The model under review builds one solid part; all positions refer to its coordinate system, in mm. Face numbers are marked on the shaded views. Round coordinates to 2 decimals unless told otherwise and drop trailing zeros. Write each loop counter-clockwise with the first axis right and the second up, starting at its lowest first coordinate (ties: lowest second). Pieces come first, ordered by that corner, then holes. Notation, with made-up numbers: (69.25, 74.5) -> (128.25, 74.5) arc R29 cw to (128.25, 101.5) -> close; hole circle Ø10 at (27, -10.5). An arc over 180 degrees is marked (long way). Use CSV: the item, a comma, the result in double quotes. Start each with the question number.
1) For pin 1 Ø12 at (y, z) = (88.5, 2) entering from -X; pin 2 Ø12 at (y, z) = (55.5, -14.5) entering from +X; pin 3 Ø10.5 at (x, z) = (40.05, -23.12) entering from -Y; pin 4 Ø12 at (y, z) = (107.5, -38.5) entering from -X, all flat-tipped, find the tip position at first contact; note any pin that passes through.
2) Take a section at C-C, the plane y = 70.5. Give the boundary of the cut face in (x, z), then the cut area to 3 significant figures.
3) Wall thickness on probe 1 along Y at (x, z) = (-24.5, -34); probe 2 along X at (y, z) = (87, 0); probe 3 along Z at (x, y) = (-36.5, 58): over which ranges is each line inside the solid? List them lowest first. Write a range as [from, to].
4) Mouldability with a two-part tool opening along Z and no side actions: class the marked faces 1, 2, 3 and 4 as released by +Z, released by -Z, zero draft, split by the parting line, or undercut.
from build123d import *

# Parameters (mm, degrees)
SKETCH1_R                       = 52.5
SKETCH1_R_2                     = 40
BOSS_EXTRUDE1_DEPTH             = 150
SKETCH7_R                       = 42.5
YLIN_URA_DEPTH                  = 3.6
SKETCH8_R                       = 42.5
TOKA_YLIN_URA_DEPTH             = 3.6
CUT_EXTRUDE5_START              = -3.6
SKETCH10_R                      = 42.5
CUT_EXTRUDE5_DEPTH              = 3.6
F_8_0MM_DOWEL_HOLE1_D           = 8
F_8_0MM_DOWEL_HOLE1_DEPTH       = 22.596557524
F_8_0MM_DOWEL_HOLE1_CSINK_D     = 8.05
F_8_0MM_DOWEL_HOLE1_CSINK_ANGLE = 90
F_8_0MM_DOWEL_HOLE1_TIP         = 2.403442476


with BuildPart() as part:
    # Sketch1 → Boss-Extrude1 (new body)
    with BuildSketch(Plane(origin=(0, 0, 0), x_dir=(1, 0, 0), z_dir=(0, 1, 0))):
        with Locations(Location((0, 0, 0), (0, 0, 270))):
            Circle(SKETCH1_R)
        with Locations(Location((0, 0, 0), (0, 0, 270))):
            Circle(SKETCH1_R_2, mode=Mode.SUBTRACT)
    extrude(amount=BOSS_EXTRUDE1_DEPTH)

    # Sketch7 → Ylin ura (cut)
    with BuildSketch(Plane(origin=(0, 135, 0), x_dir=(1, 0, 0), z_dir=(0, 1, 0))):
        with Locations(Location((0, 0, 0), (0, 0, 270))):
            Circle(SKETCH7_R)
    extrude(amount=-YLIN_URA_DEPTH, mode=Mode.SUBTRACT)

    # Sketch8 → Toka ylin ura (cut)
    with BuildSketch(Plane(origin=(0, 109.9, 0), x_dir=(1, 0, 0), z_dir=(0, 1, 0))):
        with Locations(Location((0, 0, 0), (0, 0, 270))):
            Circle(SKETCH8_R)
    extrude(amount=-TOKA_YLIN_URA_DEPTH, mode=Mode.SUBTRACT)

    # Sketch10 → Cut-Extrude5 (cut)
    with BuildSketch(Plane(origin=(0, 50.1, 0), x_dir=(-1, 0, 0), z_dir=(0, -1, 0)).offset(CUT_EXTRUDE5_START)):
        with Locations(Location((0, 0, 0), (0, 0, 270))):
            Circle(SKETCH10_R)
    extrude(amount=CUT_EXTRUDE5_DEPTH, mode=Mode.SUBTRACT)

    # Ø8.0mm Dowel Hole1
    with Locations(Plane(origin=(0, 0, 0), x_dir=(-1, 0, 0), z_dir=(0, -1, 0))):
        with Locations((0, -46.25), (-40.053674925, -23.125), (-40.053674925, 23.125), (0, 46.25), (40.053674925, 23.125), (40.053674925, -23.125)):
            CounterSinkHole(F_8_0MM_DOWEL_HOLE1_D / 2, F_8_0MM_DOWEL_HOLE1_CSINK_D / 2, depth=F_8_0MM_DOWEL_HOLE1_DEPTH, counter_sink_angle=F_8_0MM_DOWEL_HOLE1_CSINK_ANGLE)
            with Locations((0, 0, -(F_8_0MM_DOWEL_HOLE1_DEPTH + F_8_0MM_DOWEL_HOLE1_TIP / 2))):  # 118° drill point
                Cone(0, F_8_0MM_DOWEL_HOLE1_D / 2, F_8_0MM_DOWEL_HOLE1_TIP, mode=Mode.SUBTRACT)


solid = part.part
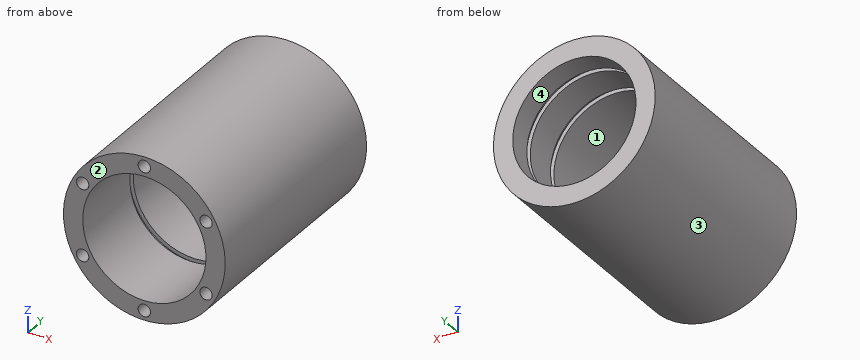
Values found:
1,pin 1,"x = -52.5"
1,pin 2,"x = 51.81"
1,pin 3,"y = 0"
1,pin 4,"x = -41.23"
2,outline,"circle Ø105 at (0, 0); hole circle Ø80 at (0, 0)"
2,area,"3,630 mm²"
3,probe 1,"[0, 50.1], [53.7, 106.3], [109.9, 131.4], [135, 150]"
3,probe 2,"[-52.5, -40], [40, 52.5]"
3,probe 3,"[-37.74, -16.36], [16.36, 37.74]"
4,face 1,"undercut"
4,face 2,"zero draft"
4,face 3,"split by the parting line"
4,face 4,"undercut"
